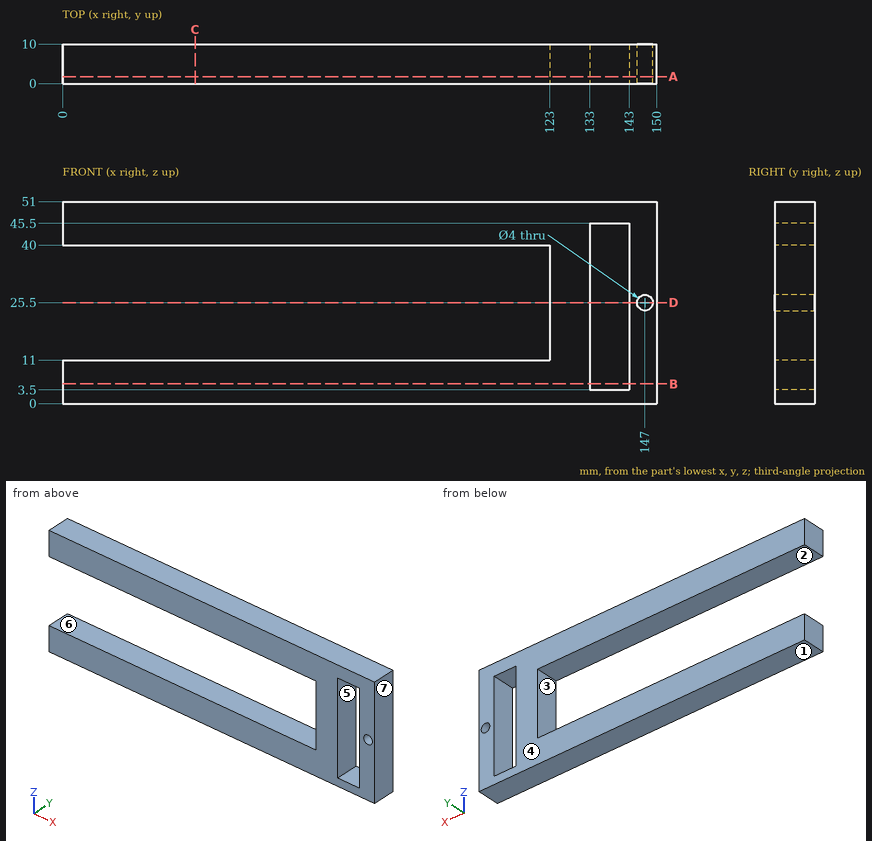
Can you work these out from the drawing? Everything is in mm from the part's minimum corner. A direction names the side the tool comes from. Round coordinates to 2 decimals unless told otherwise and drop trailing zeros. Write each loop counter-clockwise with the first axis right and the second up, starting at its lowest first coordinate (ties: lowest second). Pieces come first, ordered by that corner, then holes. Notation, with made-up numbers: (89, 88.25) - (144, 88.25) arc R19 ccw to (144, 109.25) - close; hole circle Ø4 at (26.25, 87). An arc over 180 degrees is marked (long way). Use a Markdown table: item, result.
Q1. I want a section at A-A (y = 1.75). List the corners of the cut face in (x, z) for me.
Output values:
| item | result |
|---|---|
| outline | (0, 0) - (150, 0) - (150, 51) - (0, 51) - (0, 40) - (123, 40) - (123, 11) - (0, 11) - close; hole (133, 3.5) - (143, 3.5) - (143, 45.5) - (133, 45.5) - close; hole circle Ø4 at (147, 25.5) |
Q2. I want a section at D-D (z = 25.5). List the corners of the cut face in (x, y) for me.
Output values:
| item | result |
|---|---|
| outline | (123, 0) - (133, 0) - (133, 10) - (123, 10) - close; (143, 0) - (145, 0) - (145, 10) - (143, 10) - close; (149, 0) - (150, 0) - (150, 10) - (149, 10) - close |
Q3. I want a section at B-B (z = 5). List the corners of the cut face in (x, y) for me, plus the area to 3 significant figures.
Output values:
| item | result |
|---|---|
| outline | (0, 0) - (133, 0) - (133, 10) - (0, 10) - close; (143, 0) - (150, 0) - (150, 10) - (143, 10) - close |
| area | 1,400 mm2 |
Q4. I want a section at C-C (x = 33.5). List the corners of the cut face in (y, z) for me, plus the area to 3 significant figures.
Output values:
| item | result |
|---|---|
| outline | (0, 0) - (10, 0) - (10, 11) - (0, 11) - close; (0, 40) - (10, 40) - (10, 51) - (0, 51) - close |
| area | 220 mm2 |
Q5. Thinking about a two-plate mould opening in Z: for the marked faces 1, 2, 3 and 4, which applies, released by +Z, released by -Z, zero draft, split by the parting line, or undercut?
Output values:
| item | result |
|---|---|
| face 1 | released by -Z |
| face 2 | undercut |
| face 3 | undercut |
| face 4 | zero draft |
Q6. For pin 1 (5 mm diameter, centred on y = 5.5, z = 20.5, fed in from -X); pin 2 (2.5 mm diameter, centred on x = 147, z = 25.5, fed in from -Y), each with a flat end and sliding along its axis, tell me the tip position at first contact or that it passes through.
Output values:
| item | result |
|---|---|
| pin 1 | x = 123 |
| pin 2 | through |
Q7. Please list where these lines run through material, in increasing order: L1, parallel to X at y = 5.75, z = 25.5; L2, parallel to X at y = 4, z = 39; L3, parallel to Z at x = 92, y = 2.
Output values:
| item | result |
|---|---|
| L1 | 123 to 133, 143 to 145, 149 to 150 |
| L2 | 123 to 133, 143 to 150 |
| L3 | 0 to 11, 40 to 51 |
Q8. For the marked faces 5, 6 and 7, which set-ups out of +Z, -Z, +X, -X, +Y, -Y let a thin tool reach every point of the face, with its end or its side?
Output values:
| item | result |
|---|---|
| face 5 | +Y, -Y |
| face 6 | -X, +Y, -Y |
| face 7 | +Z, -Z, +X, +Y, -Y |
